Could you check a few things on this drawing? It's one solid part, dimensions in mm from its lowest x, y, z. Round coordinates to 2 decimals unless told otherwise and drop trailing zeros. Order: outer loops, then holes, each group sorted by start corner. A loop starts at its lowest first (then second) coordinate and runs counter-clockwise, first axis right, second up. Notation, with made-up numbers: M 1.25,30.5 L 23.25,30.5 A31 cw 23.25,54.5 Z; hole C -16,-18 d8. An arc over 180 degrees is marked long. Answer as CSV lines item,"result". Start each with the question number.
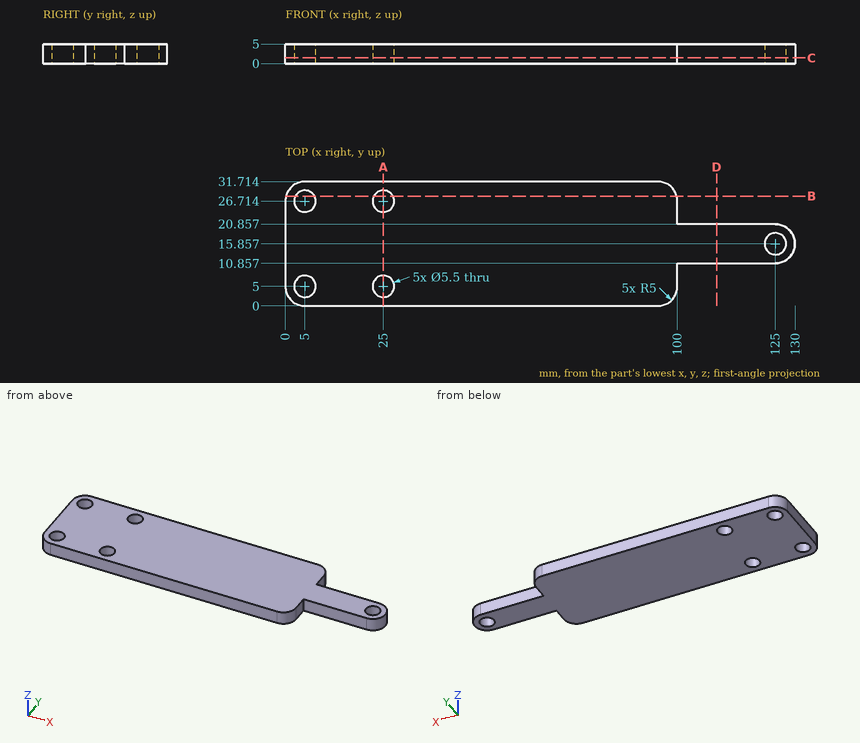
Item 1: If we section it at C-C on z = 1.45: Please give me the cut outline in (x, y), and give its area (3 significant figures).
Item 2: If we section it at A-A on x = 25: Please give me the cut outline in (y, z), and give its area (3 significant figures).
Item 3: For P1, Ø1, axis at y = 3.5, z = 0.5, coming from the +X side; P2, Ø1.5, axis at y = 22.5, z = 1.5, coming from the +X side; P3, Ø2.5, axis at x = 112.5, z = 3, coming from the -Y side, each with a flat end and sliding along its axis, tell me the tip position at first contact or that it passes through.
Item 4: If I drill on line 1 along Y through (x, z) = (5, 2.5); line 2 along X through (y, z) = (27, 1.7); line 3 along Y through (x, z) = (125, 2.8), over which ranges is the centre line in solid material (lowest first)?
Item 5: If we section it at B-B on y = 28: Please give me the cut outline in (x, z), and give its area (3 significant figures).
Item 6: If we section it at D-D on x = 110: Please give me the cut outline in (y, z), and give its area (3 significant figures).
Geometry says:
1,outline,"M 0,5 A5 ccw 5,0 L 95,0 A5 ccw 100,5 L 100,10.86 L 125,10.86 A5 ccw 125,20.86 L 100,20.86 L 100,26.71 A5 ccw 95,31.71 L 5,31.71 A5 ccw 0,26.71 Z; hole C 5,5 d5.5; hole C 5,26.71 d5.5; hole C 25,5 d5.5; hole C 25,26.71 d5.5; hole C 125,15.86 d5.5"
1,area,"3,320 mm²"
2,outline,"M 0,0 L 2.25,0 L 2.25,5 L 0,5 Z; M 7.75,0 L 23.96,0 L 23.96,5 L 7.75,5 Z; M 29.46,0 L 31.71,0 L 31.71,5 L 29.46,5 Z"
2,area,"104 mm²"
3,P1,"x = 99.9"
3,P2,"x = 100"
3,P3,"y = 10.86"
4,line 1,"0 to 2.25, 7.75 to 23.96, 29.46 to 31.71"
4,line 2,"0.01 to 2.26, 7.74 to 22.26, 27.74 to 99.99"
4,line 3,"10.86 to 13.11, 18.61 to 20.86"
5,outline,"M 0.17,0 L 2.57,0 L 2.57,5 L 0.17,5 Z; M 7.43,0 L 22.57,0 L 22.57,5 L 7.43,5 Z; M 27.43,0 L 99.83,0 L 99.83,5 L 27.43,5 Z"
5,area,"450 mm²"
6,outline,"M 10.86,0 L 20.86,0 L 20.86,5 L 10.86,5 Z"
6,area,"50.0 mm²"
